```python
from build123d import *

# Parameters (mm, degrees)
CROQUIS1_W              = 22
CROQUIS1_H              = 10.65
SALIENTE_EXTRUIR1_DEPTH = 74
CORTAR_EXTRUIR1_REACH   = 12.65
CROQUIS2_R              = 3.25


with BuildPart() as part:
    # Croquis1 → Saliente-Extruir1 (new body)
    with BuildSketch(Plane.XY):
        with Locations((18, 0)):
            Rectangle(CROQUIS1_W, CROQUIS1_H)
    extrude(amount=SALIENTE_EXTRUIR1_DEPTH)

    # Croquis2 → Cortar-Extruir1 (cut, up to next)
    with BuildSketch(Plane(origin=(0, 5.325, 0), x_dir=(1, 0, 0), z_dir=(0, 1, 0)), mode=Mode.PRIVATE) as cortar_extruir1_sk1:
        with Locations((18, -7)):
            Circle(CROQUIS2_R)
    cortar_extruir1_tool1 = extrude(cortar_extruir1_sk1.sketch, amount=-CORTAR_EXTRUIR1_REACH, mode=Mode.PRIVATE) & part.part
    add(cortar_extruir1_tool1.solids().sort_by_distance((18, 5.325, 7))[0], mode=Mode.SUBTRACT)
    # Croquis2 → Cortar-Extruir1 (cut, up to next)
    with BuildSketch(Plane(origin=(0, 5.325, 0), x_dir=(1, 0, 0), z_dir=(0, 1, 0)), mode=Mode.PRIVATE) as cortar_extruir1_sk2:
        with Locations((18, -67)):
            Circle(CROQUIS2_R)
    cortar_extruir1_tool2 = extrude(cortar_extruir1_sk2.sketch, amount=-CORTAR_EXTRUIR1_REACH, mode=Mode.PRIVATE) & part.part
    add(cortar_extruir1_tool2.solids().sort_by_distance((18, 5.325, 67))[0], mode=Mode.SUBTRACT)


solid = part.part
```
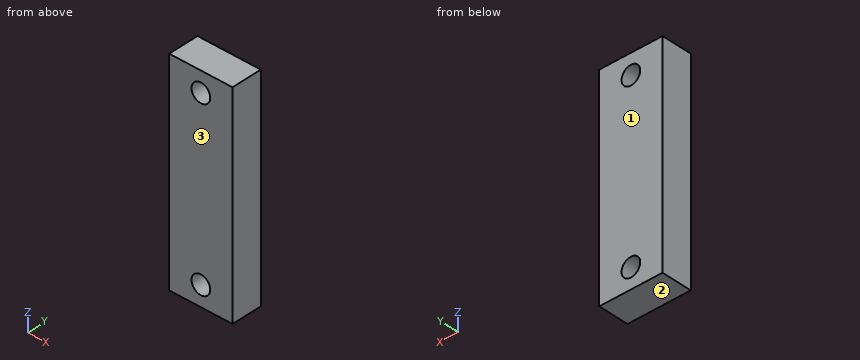
Can you work these out from the model? Positions are in its coordinate system, mm. Face numbers are marked on the shaded views. Round coordinates to 2 decimals unless told otherwise and drop trailing zeros. Loops run counter-clockwise (first coordinate to the right, second up) from the corner with the lowest first, then second, coordinate; pieces in that order, holes last. Notation, with made-up numbers: (34.5, 45.25) -> (90.5, 45.25) arc R17 cw to (90.5, 69.25) -> close; hole circle Ø11 at (74.25, 51). An arc over 180 degrees is marked (long way). One line per item, written item: value. Start each with the question number.
1. If I drill on probe 1 along Z at (x, y) = (18, -2.25); probe 2 along Z at (x, y) = (16.75, -1.75); probe 3 along X at (y, z) = (-2.25, 7), over which ranges is the centre line in solid material (lowest first)?
2. If we section it at C-C, the plane y = 3.5: Write out the boundary of the cut face in (x, z).
3. For pin 1 (6 mm diameter, centred on x = 18, z = 7, fed in from -Y), with a flat end and sliding along its axis, tell me the tip position at first contact or that it passes through.
4. If we section it at B-B, the plane z = 67: Write out the boundary of the cut face in (x, y) (3 decimals), then the cut area to 3 significant figures.
5. If we mould it in two halves opening along Y, with no side actions, what happens to the marked faces 1, 2 and 3? For each: pulls with the +Y half, pulls with the -Y half, needs draft (parallel to the pull), parting line crosses it, or undercut.
6. If we section it at A-A, the plane x = 18: Write out the boundary of the cut face in (y, z) (3 decimals).
Calculated:
1. probe 1: z = 0 to 3.75, 10.25 to 63.75, 70.25 to 74
1. probe 2: z = 0 to 4, 10 to 64, 70 to 74
1. probe 3: x = 7 to 14.75, 21.25 to 29
2. outline: (7, 0) -> (29, 0) -> (29, 74) -> (7, 74) -> close; hole circle Ø6.5 at (18, 7); hole circle Ø6.5 at (18, 67)
3. pin 1: passes through
4. outline: (7, -5.325) -> (14.75, -5.325) -> (14.75, 5.325) -> (7, 5.325) -> close; (21.25, -5.325) -> (29, -5.325) -> (29, 5.325) -> (21.25, 5.325) -> close
4. area: 165 mm²
5. face 1: pulls with the +Y half
5. face 2: needs draft
5. face 3: pulls with the -Y half
6. outline: (-5.325, 0) -> (5.325, 0) -> (5.325, 3.75) -> (-5.325, 3.75) -> close; (-5.325, 10.25) -> (5.325, 10.25) -> (5.325, 63.75) -> (-5.325, 63.75) -> close; (-5.325, 70.25) -> (5.325, 70.25) -> (5.325, 74) -> (-5.325, 74) -> close
